Geometry: final body of the model. Coordinates: model frame, mm. A direction names the side the tool comes from. Give positions to 0.01 mm unless a question says otherwise; leave off trailing zeros. Loops run counter-clockwise (first coordinate to the right, second up) from the corner with the lowest first, then second, coordinate; pieces in that order, holes last. Notation, with made-up numbers: M 55,2 L 75,2 A26 ccw 75,28 Z; hole C 57,31.5 d7. An arc over 180 degrees is marked long. Put each result on its own line as item: value.
```python
from build123d import *

# Parameters (mm, degrees)
SKETCH_1_R               = 30
EXTRUDE_1_DEPTH          = 6
EXTRUDE_START            = 6
SKETCH_3_R               = 19
EXTRUDE_2_DEPTH          = 1
EXTRUDE_START_2          = 7
SKETCH_4_R               = 17.5
EXTRUDE_3_DEPTH          = 20
SKETCH_5_R               = 15.1
CUT_EXTRUDE_1_DEPTH      = 5
SKETCH_6_R               = 1.75
CUT_EXTRUDE_2_DEPTH      = 51.289163843
PATTERN_CIRCULAR_1_COUNT = 3
SKETCH1_R                = 3.25
CUT_EXTRUDE1_DEPTH       = 14
CUT_EXTRUDE_3_DEPTH      = 51.289163843
CUT_EXTRUDE_3_DEPTH_BACK = 51.289163843
SKETCH_7_R               = 1.25
SKETCH_8_R               = 1.75
CUT_EXTRUDE_4_DEPTH      = 51.289163843
CUT_EXTRUDE_START        = 3
CUT_EXTRUDE_5_DEPTH      = 10
PATTERN_CIRCULAR_2_COUNT = 4
CHAMFER2_SIZE            = 0.5
CHAMFER1_SIZE            = 0.5


with BuildPart() as part:
    # Sketch 1 → Extrude 1 (new body)
    with BuildSketch(Plane(origin=(0, 0, 0), x_dir=(1, 0, 0), z_dir=(0, 1, 0))):
        with Locations(Location((0, 0, 0), (0, 0, 270))):
            Circle(SKETCH_1_R)
    extrude(amount=EXTRUDE_1_DEPTH)

    # Sketch 3 → Extrude 2 (add)
    with BuildSketch(Plane(origin=(0, 0, 0), x_dir=(1, 0, 0), z_dir=(0, 1, 0)).offset(EXTRUDE_START)):
        with Locations(Location((0, 0, 0), (0, 0, 270))):
            Circle(SKETCH_3_R)
    extrude(amount=EXTRUDE_2_DEPTH)

    # Sketch 4 → Extrude 3 (add)
    with BuildSketch(Plane(origin=(0, 0, 0), x_dir=(1, 0, 0), z_dir=(0, 1, 0)).offset(EXTRUDE_START_2)):
        with Locations(Location((0, 0, 0), (0, 0, 270))):
            Circle(SKETCH_4_R)
    extrude(amount=EXTRUDE_3_DEPTH)

    # Sketch 5 → Cut-Extrude 1 (cut)
    with BuildSketch(Plane(origin=(0, 27, 0), x_dir=(1, 0, 0), z_dir=(0, 1, 0))):
        with Locations(Location((0, 0, 0), (0, 0, 270))):
            Circle(SKETCH_5_R)
    extrude(amount=-CUT_EXTRUDE_1_DEPTH, mode=Mode.SUBTRACT)

    # Sketch 6 → Cut-Extrude 2 (cut, through all)
    with BuildSketch(Plane(origin=(0, 0, 0), x_dir=(1, 0, 0), z_dir=(0, 1, 0))):
        with Locations(Location((0, 12, 0), (0, 0, 270))):
            Circle(SKETCH_6_R)
    cut_extrude_2 = extrude(amount=CUT_EXTRUDE_2_DEPTH, mode=Mode.SUBTRACT)

    # Pattern Circular 1: Cut-Extrude 2 ×3 about axis
    pattern_circular_1_axis = Axis((0, 0, 0), (0, 1, 0))
    for i in range(1, PATTERN_CIRCULAR_1_COUNT):
        add(cut_extrude_2.rotate(pattern_circular_1_axis, i * 360 / PATTERN_CIRCULAR_1_COUNT), mode=Mode.SUBTRACT)

    # Sketch1 → Cut-Extrude1 (cut)
    with BuildSketch(Plane.XZ):
        with Locations(Location((-10.392304845, 6, 0), (0, 0, 270))):
            Circle(SKETCH1_R)
        with Locations(Location((10.392304845, 6, 0), (0, 0, 270))):
            Circle(SKETCH1_R)
        with Locations(Location((0, -12, 0), (0, 0, 270))):
            Circle(SKETCH1_R)
    extrude(amount=-CUT_EXTRUDE1_DEPTH, mode=Mode.SUBTRACT)

    # Sketch 7 → Cut-Extrude 3 (cut, two sides: drawn at the far end of the back side and taken through both)
    with BuildSketch(Plane.XZ.offset(-CUT_EXTRUDE_3_DEPTH_BACK)):
        with Locations(Location((0, 0, 0), (0, 0, 90))):
            Circle(SKETCH_7_R)
    extrude(amount=CUT_EXTRUDE_3_DEPTH + CUT_EXTRUDE_3_DEPTH_BACK, mode=Mode.SUBTRACT)

    # Sketch 8 → Cut-Extrude 4 (cut, through all)
    with BuildSketch(Plane(origin=(0, 0, 0), x_dir=(1, 0, 0), z_dir=(0, 1, 0))):
        with Locations(Location((17.039195094, 16.901651711, 0), (0, 0, 270))):
            Circle(SKETCH_8_R)
    cut_extrude_4 = extrude(amount=CUT_EXTRUDE_4_DEPTH, mode=Mode.SUBTRACT)

    # Sketch 8_3 → Cut-Extrude 5 (cut)
    with BuildSketch(Plane(origin=(0, 0, 0), x_dir=(1, 0, 0), z_dir=(0, 1, 0)).offset(CUT_EXTRUDE_START)):
        Polygon((14.712179838, 14.574636455), (17.890941793, 13.722889756), (20.217957048, 16.049905012), (19.36621035, 19.228666966), (16.187448396, 20.080413665), (13.86043314, 17.753398409), align=None)
    cut_extrude_5 = extrude(amount=CUT_EXTRUDE_5_DEPTH, mode=Mode.SUBTRACT)

    # Pattern Circular 2: Cut-Extrude 4, Cut-Extrude 5 ×4 about axis
    pattern_circular_2_axis = Axis((0, 0, 0), (0, 1, 0))
    add([cut_extrude_4.rotate(pattern_circular_2_axis, i * 360 / PATTERN_CIRCULAR_2_COUNT) for i in range(1, PATTERN_CIRCULAR_2_COUNT)], mode=Mode.SUBTRACT)
    add([cut_extrude_5.rotate(pattern_circular_2_axis, i * 360 / PATTERN_CIRCULAR_2_COUNT) for i in range(1, PATTERN_CIRCULAR_2_COUNT)], mode=Mode.SUBTRACT)

    # Chamfer2
    chamfer2_edges = [part.edges().sort_by_distance(p)[0] for p in [
        (0, 0, -30),
        (0, 6, -30),
    ]]
    chamfer(chamfer2_edges, length=CHAMFER2_SIZE)

    # Chamfer1
    chamfer1_edges = [part.edges().sort_by_distance(p)[0] for p in [
        (0, 27, -17.5),
        (0, 0, -1.25),
        (0, 22, -1.25),
    ]]
    chamfer(chamfer1_edges, length=CHAMFER1_SIZE)


solid = part.part
```
Item 1: Mould query, pull axis Z, two halves, no side actions, for faces 4 (the flat face through (0.4, 6, 19.3)), 5 (the cylindrical face through (-18.774, 1.479, 17.129)). Classes: pulls with the +Z half, pulls with the -Z half, needs draft (parallel to the pull), parting line crosses it, or undercut.
Output values:
face 4: needs draft
face 5: undercut
Item 2: Section A-A on x = 0. Count the separate pieces of the cut face and the enclosed holes in it, then the cut area to 3 significant figures.
Output values:
separate pieces: 3
enclosed holes: 0
area: 772 mm²
Item 3: Set-up query: faces 1 (the flat face through (-18.933, 4.479, -15.04)), 2 (the flat face through (-11.8, 14, 4.6)), 3 (the cylindrical face through (1.22, 11.15, -0.27)). Return all of +Z, -Z, +X, -X, +Y, -Y with unobstructed straight access to the full face (end or side cutting, diameter ignored); none if empty.
Output values:
face 1: +Y
face 2: -Y
face 3: +Y, -Y
Item 4: Pin query (flat end, axial travel): pin 1 Ø8 at (x, y) = (-12.5, 16.5) entering from -Z; pin 2 Ø2 at (x, y) = (-3.5, 13) entering from +Z; pin 3 Ø10 at (y, z) = (12, 12) entering from +X; pin 4 Ø2 at (x, z) = (0, -12) entering from +Y. Return the tip coordinate at first contact, or that it passes through.
Output values:
pin 1: z = -15.3
pin 2: z = 17.32
pin 3: x = 16.04
pin 4: through
Item 5: Section B-B on y = 17.5. Output: boundary loops of the cut face in (x, z) (3 decimals).
Output values:
outline: C 0,0 d35; hole C -10.392,6 d3.5; hole C 0,-12 d3.5; hole C 0,0 d2.5; hole C 10.392,6 d3.5
Item 6: Line query: probe 1 along X at (y, z) = (15.5, 0); probe 2 along Z at (x, y) = (18.5, 2); probe 3 along Y at (x, z) = (7.5, 21). Output: solid intervals per line, ascending. Write a range as [from, to].
Output values:
probe 1: [-17.5, -1.25], [1.25, 17.5]
probe 2: [-23.62, -17.87], [-15.94, 16.33], [17.75, 23.62]
probe 3: [0, 6]
